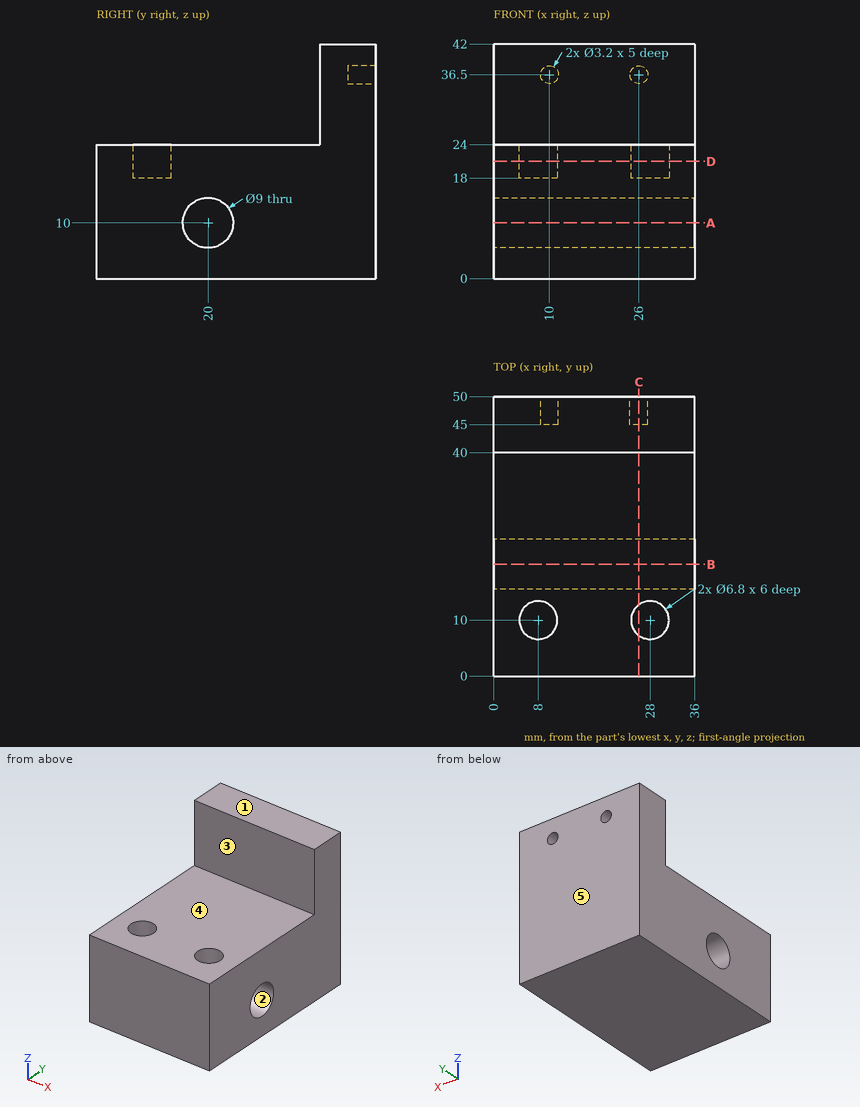
The drawing under review shows one solid part. Ordinate dimensions are in mm from its lowest x, y, z. A direction names the side the tool comes from. Coordinates: 2 decimals unless noted, no trailing zeros. Write each loop counter-clockwise with the first axis right and the second up, starting at its lowest first coordinate (ties: lowest second). Pieces come first, ordered by that corner, then holes. Notation, with made-up numbers: (-19.75, 40.5) - (14.25, 40.5) arc R18 cw to (14.25, 53.5) - close; hole circle Ø1 at (72.25, 14). An arc over 180 degrees is marked (long way). Put each result on its own line as item: value.
1. Add section C-C, the plane x = 26. Give the boundary of the cut face in (y, z).
Values found:
outline: (0, 0) - (50, 0) - (50, 34.9) - (45, 34.9) - (45, 38.1) - (50, 38.1) - (50, 42) - (40, 42) - (40, 24) - (12.75, 24) - (12.75, 18) - (7.25, 18) - (7.25, 24) - (0, 24) - close; hole circle Ø9 at (20, 10)
2. Add section D-D, the plane z = 21. Give the boundary of the cut face in (x, y).
Values found:
outline: (0, 0) - (36, 0) - (36, 50) - (0, 50) - close; hole circle Ø6.8 at (8, 10); hole circle Ø6.8 at (28, 10)
3. Add section A-A, the plane z = 10. Give the boundary of the cut face in (x, y).
Values found:
outline: (0, 0) - (36, 0) - (36, 15.5) - (0, 15.5) - close; (0, 24.5) - (36, 24.5) - (36, 50) - (0, 50) - close
4. Wall thickness on probe 1 along Y at (x, z) = (16.5, 10); probe 2 along Y at (x, z) = (28, 21); probe 3 along Y at (x, z) = (27, 28): over which ranges is each line inside the solid? List them lowest first.
Values found:
probe 1: 0 to 15.5, 24.5 to 50
probe 2: 0 to 6.6, 13.4 to 50
probe 3: 40 to 50
5. Mouldability with a two-part tool opening along Y and no side actions: class the marked faces 1, 2 and 3 as released by +Y, released by -Y, zero draft, split by the parting line, or undercut.
Values found:
face 1: zero draft
face 2: undercut
face 3: released by -Y
6. Add section B-B, the plane y = 20. Give the boundary of the cut face in (x, z), then the cut area to 3 significant figures.
Values found:
outline: (0, 0) - (36, 0) - (36, 5.5) - (0, 5.5) - close; (0, 14.5) - (36, 14.5) - (36, 24) - (0, 24) - close
area: 540 mm²
7. Machinability: for the marked faces 4 and 5, which of the approach directions +Z, -Z, +X, -X, +Y, -Y give a long, thin tool a straight path to every point of the face, cutting with its end or side? Answer none if there is none.
Values found:
face 4: +Z, +X, -X, -Y
face 5: +Z, -Z, +X, -X, +Y
8. For pin 1 (3 mm diameter, centred on x = 10, z = 36.5, fed in from +Y); pin 2 (2 mm diameter, centred on x = 6.5, y = 9, fed in from +Z); pin 3 (5.5 mm diameter, centred on x = 28.5, y = 11.5, fed in from +Z), all flat-tipped, find the tip position at first contact; note any pin that passes through.
Values found:
pin 1: y = 45
pin 2: z = 18
pin 3: z = 24
